Here's how the part is built. I have some questions about the finished solid (model axes, mm). Face numbers are marked on the shaded views. A direction names the side the tool comes from. Round coordinates to 2 decimals unless told otherwise and drop trailing zeros. Write each loop counter-clockwise with the first axis right and the second up, starting at its lowest first coordinate (ties: lowest second). Pieces come first, ordered by that corner, then holes. Notation, with made-up numbers: (-26.5, 26.25) -> (-7.5, 26.25) arc R14 cw to (-7.5, 43.25) -> close; hole circle Ø10 at (59.25, 19). An arc over 180 degrees is marked (long way). Put each result on its own line as item: value. Start each with the question number.
1. I need wall thicknesses on probe 1 along Y at (x, z) = (0.75, 2.5); probe 2 along Y at (x, z) = (-0.5, -2); probe 3 along Y at (x, z) = (-3.25, -0.25). Which ranges of each line are inside material? Lowest first, please. Write a range as from..to.
2. Suppose I cut it at B-B (x = -2.25). Please give me the cut outline in (y, z).
3. Suppose I cut it at C-C (y = 5.25). Please give me the cut outline in (x, z).
4. We'd pull the mould along Z, two halves only. Please class the marked faces 5, 6 and 7: +Z half, -Z half, draft (parallel to the pull), parting line (faces both ways), or undercut.
5. Suppose I cut it at D-D (y = 10.75). Please give me the cut outline in (x, z), then the cut area to 3 significant figures.
6. For pin 1 (1.5 mm diameter, centred on x = 3, z = -2, fed in from +Y); pin 2 (1.6 mm diameter, centred on x = 0, z = 0, fed in from +Y); pin 3 (2 mm diameter, centred on x = 1.5, z = 1, fed in from -Y); pin 4 (2 mm diameter, centred on y = 4, z = 1.5, fed in from -X), each with a flat end and sliding along its axis, tell me the tip position at first contact or that it passes through.
7. Which directions (+Z, -Z, +X, -X, +Y, -Y) give clear straight access to the entire face, cutting with the end or side of a thin tool? Please do the marked faces 1, 2, 3 and 4.
8. Suppose I cut it at A-A (y = 2.5). Please give me the cut outline in (x, z).
Autodesk Inventor part; units mm, degrees
ref_plane "YZ Plane" through (0, 0, 0) normal (1, 0, 0) x (0, 1, 0)
ref_plane "XZ Plane" through (0, 0, 0) normal (0, 1, 0) x (-1, 0, 0)
ref_plane "XY Plane" through (0, 0, 0) normal (0, 0, 1) x (1, 0, 0)
sketch "Sketch1" plane through (0, 0, 0) normal (0, 0, 1) x (1, 0, 0)
  line L0 (0, 0) -> (0.5, 0)
  line L1 (0.5, 0) -> (1.9004, 2)
  line L2 (1.9004, 2) -> (7, 2)
  line L3 (7, 2) -> (7, 5)
  line L4 (7, 5) -> (2.5, 5)
  line L5 (2.5, 5) -> (2.5, 6.5)
  line L6 (2.5, 6.5) -> (3, 6.5)
  line L7 (3, 6.5) -> (3, 12.5)
  line L8 (3, 12.5) -> (0, 12.5)
  line L9 (0, 12.5) -> (0, 0)
  dimension "d0" = 0.5
  dimension "d1" = 125
  dimension "d2" = 6
  dimension "d3" = 7.5
  dimension "d4" = 10.5
  dimension "d5" = 12.5
  dimension "d6" = 3
  dimension "d7" = 2.5
  dimension "d8" = 7
revolve "Revolution1" add sketch "Sketch1" angle 360 about axis through (0, 12.5, 0) along (0, -1, 0)
sketch "Sketch2" plane through (0, 2, 0) normal (0, -1, 0) x (1, 0, 0)
  circle A0 centre (0, 0) radius 2.5
  circle A1 centre (0, 0) radius 7
  circle A2 centre (0, 0) radius 0.5
  line L0 (2.0207, 3.5) -> (4.0415, 0)
  line L1 (4.0415, 0) -> (2.0207, -3.5)
  line L2 (2.0207, -3.5) -> (-2.0207, -3.5)
  line L3 (-2.0207, -3.5) -> (-4.0415, 0)
  line L4 (-4.0415, 0) -> (-2.0207, 3.5)
  line L5 (-2.0207, 3.5) -> (2.0207, 3.5)
  point P0 (0, 0)
  dimension "d10" = 7
  dimension "d11" = 3.5
extrude "Extrusion1" cut sketch "Sketch2" against normal blind 10 contours A1
thread "Thread1"
hole "Hole1" at (0, 12.5, 0) direction (0, -1, 0) diameter 2 depth 10.5 tip angle 118
hole "Hole2" at (0, 12.5, 0) direction (0, -1, 0) diameter 0.5 end through all
hole "Hole3" at (0, 12.5, 0) direction (0, -1, 0) diameter 1.5 depth 11.5 tip angle 118
properties part number "Nozzle" material "Brass, Soft Yellow"
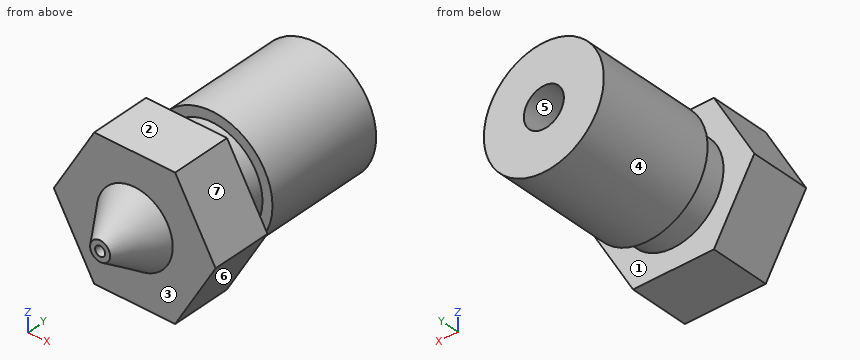
Verdict:
1. probe 1: y = 2..5, 6.5..12.5
1. probe 2: y = 2..12.5
1. probe 3: y = 2..5
2. outline: (2, -3.1) -> (5, -3.1) -> (5, -1.09) -> (6.5, -1.09) -> (6.5, -1.98) -> (12.5, -1.98) -> (12.5, 1.98) -> (6.5, 1.98) -> (6.5, 1.09) -> (5, 1.09) -> (5, 3.1) -> (2, 3.1) -> close
3. outline: circle Ø5 at (0, 0); hole circle Ø2 at (0, 0)
4. face 5: undercut
4. face 6: -Z half
4. face 7: +Z half
5. outline: circle Ø6 at (0, 0); hole circle Ø2 at (0, 0)
5. area: 25.1 mm^2
6. pin 1: stops at y = 12.5
6. pin 2: stops at y = 1.88
6. pin 3: stops at y = 0.43
6. pin 4: stops at x = -3.75
7. face 1: none
7. face 2: +Z, +X, -X, +Y, -Y
7. face 3: -Y
7. face 4: +Y
8. outline: (-4.04, 0) -> (-2.02, -3.5) -> (2.02, -3.5) -> (4.04, 0) -> (2.02, 3.5) -> (-2.02, 3.5) -> close; hole circle Ø2 at (0, 0)
